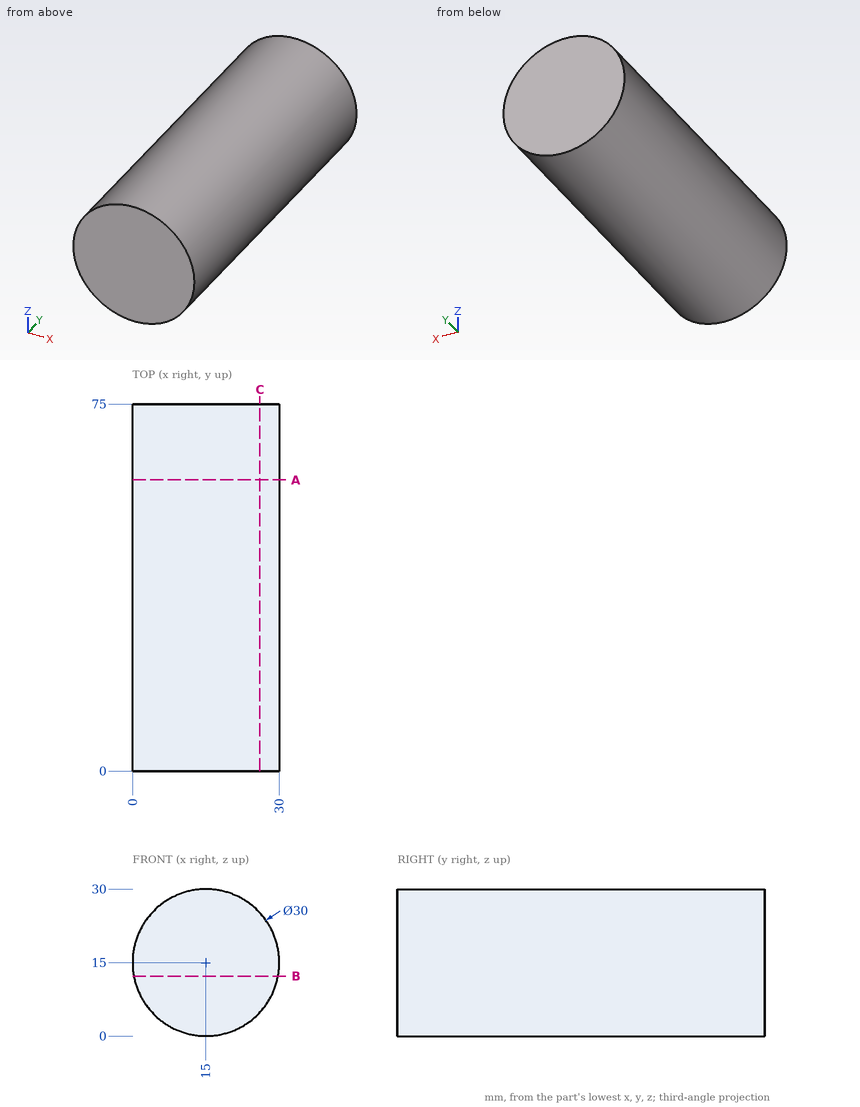
Design review of the part shown in the three views and the two pictorial views. Dimensions are in mm from the part's minimum x, y and z. Give positions to 0.01 mm unless a question says otherwise; leave off trailing zeros. Write each loop counter-clockwise with the first axis right and the second up, starting at its lowest first coordinate (ties: lowest second). Pieces come first, ordered by that corner, then holes. Notation, with made-up numbers: M 12,25 L 50,25 A28 cw 50,45 Z; hole C -21,19.25 d1. An arc over 180 degrees is marked long. One line per item, written item: value.
1) For P1, Ø12, axis at x = 16, y = 41, coming from the +Z side; P2, Ø6, axis at x = 10, y = 10.5, coming from the -Z side; P3, Ø2, axis at y = 52, z = 6.5, coming from the +X side; P4, Ø4, axis at x = 25, y = 9.5, coming from the +Z side, all flat-tipped, find the tip position at first contact; note any pin that passes through.
Results are:
P1: stops at z = 30
P2: stops at z = 0.13
P3: stops at x = 27.99
P4: stops at z = 27.69
2) Take a section at A-A, the plane y = 59.5. Write out the cut boundary in (x, z), then the cut area to 3 significant figures.
Results are:
outline: C 15,15 d30
area: 707 mm²
3) Take a section at B-B, the plane z = 12.25. Write out the cut boundary in (x, y), then the cut area to 3 significant figures.
Results are:
outline: M 0.25,0 L 29.75,0 L 29.75,75 L 0.25,75 Z
area: 2,210 mm²
4) Take a section at C-C, the plane x = 26. Write out the cut boundary in (y, z), then the cut area to 3 significant figures.
Results are:
outline: M 0,4.8 L 75,4.8 L 75,25.2 L 0,25.2 Z
area: 1,530 mm²
5) For line 1 (X direction, y = 65.5, z = 14.5); line 2 (Z direction, x = 14.75, y = 16); line 3 (X direction, y = 9, z = 9), list the stretches that pass through material, from the lowest coordinate up. Write a range as from..to.
Results are:
line 1: x = 0.01..29.99
line 2: z = 0..30
line 3: x = 1.25..28.75
